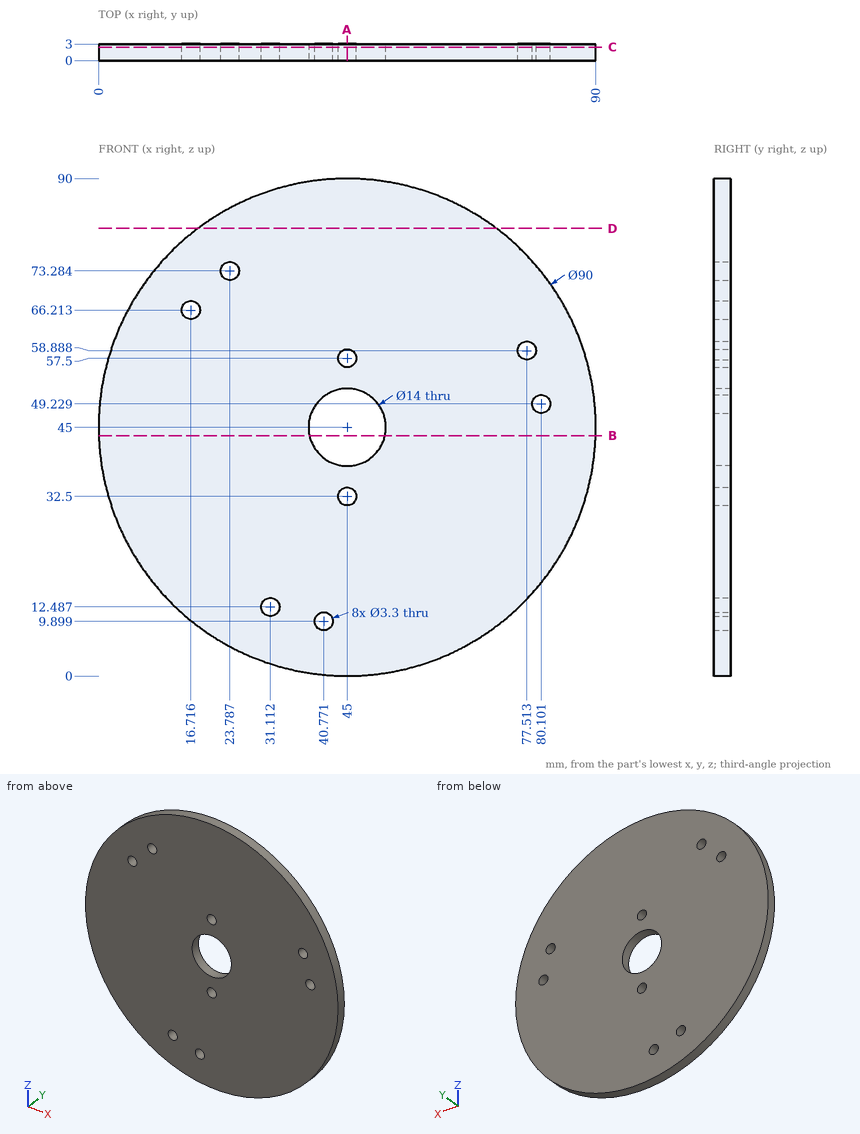
Verification items for this drawing (mm, ordinates from the low corner). Give positions to 0.01 mm unless a question says otherwise; leave off trailing zeros. Loops run counter-clockwise (first coordinate to the right, second up) from the corner with the lowest first, then second, coordinate; pieces in that order, holes last. Notation, with made-up numbers: M -5.5,14 L 3.5,14 A15 cw 3.5,32 Z; hole C -29.5,65.5 d1. An arc over 180 degrees is marked long. Answer as CSV lines item,"result".
Item 1: Cross-section at D-D on z = 81. Record the cut outline in (x, y), and give its area (3 significant figures).
Values:
outline,"M 18,0 L 72,0 L 72,3 L 18,3 Z"
area,"162 mm²"
Item 2: Cross-section at B-B on z = 43.5. Record the cut outline in (x, y) (1 decimal), and give its area (3 significant figures).
Values:
outline,"M 0,0 L 38.2,0 L 38.2,3 L 0,3 Z; M 51.8,0 L 90,0 L 90,3 L 51.8,3 Z"
area,"229 mm²"
Item 3: Material ranges on line 1 (Z direction, x = 45, y = 2.5); line 2 (Z direction, x = 43.5, y = 2.45) (1 decimal); line 3 (Z direction, x = 40, y = 2.95) (1 decimal), recorded low to high.
Values:
line 1,"z = 0 to 30.85, 34.15 to 38, 52 to 55.85, 59.15 to 90"
line 2,"z = 0 to 31.8, 33.2 to 38.2, 51.8 to 56.8, 58.2 to 90"
line 3,"z = 0.3 to 8.4, 11.4 to 40.1, 49.9 to 89.7"
Item 4: Cross-section at C-C on y = 2.45. Count the separate pieces of the cut face and the enclosed holes in it, and give its area (3 significant figures).
Values:
separate pieces,"1"
enclosed holes,"9"
area,"6,140 mm²"
Item 5: Cross-section at A-A on x = 45. Record the cut outline in (y, z), and give its area (3 significant figures).
Values:
outline,"M 0,0 L 3,0 L 3,30.85 L 0,30.85 Z; M 0,34.15 L 3,34.15 L 3,38 L 0,38 Z; M 0,52 L 3,52 L 3,55.85 L 0,55.85 Z; M 0,59.15 L 3,59.15 L 3,90 L 0,90 Z"
area,"208 mm²"
Item 6: Depth check by flat-ended pin: P1, Ø1, axis at x = 11.5, y = 1, coming from the -Z side (1 decimal); P2, Ø3, axis at x = 45, z = 57.5, coming from the -Y side. Enter the tip coordinate at first touch or a pass-through.
Values:
P1,"stops at z = 14.4"
P2,"passes through"
